```python
from build123d import *

# Parameters (mm, degrees)
ESQUISSE1_R                               = 30
BOSS_EXTRU_1_DEPTH                        = 5
ESQUISSE6_R                               = 35
ESQUISSE6_R_2                             = 30
BOSS_EXTRU_6_DEPTH                        = 5
ESQUISSE7_R                               = 32.5
ESQUISSE7_R_2                             = 30
BOSS_EXTRU_8_DEPTH                        = 35
CONG_2_R                                  = 10
BOSS_EXTRU_9_DEPTH                        = 30
BOSS_EXTRU_10_DEPTH                       = 12
CHANFREIN1_SIZE                           = 6
CONG_3_R                                  = 5
ENL_V_MAT_EXTRU_1_REACH                   = 89.234
ENL_V_MAT_EXTRU_1_END_RADIUS              = 32.5
ESQUISSE10_R                              = 4.5
ESQUISSE11_R                              = 4.5
ESQUISSE11_R_2                            = 2.6
BOSS_EXTRU_11_DEPTH                       = 3
R_P_TITION_CIRCULAIRE1_COUNT              = 4
CHANFREIN1_OF_R_P_TITION_CIRCULAIRE1_SIZE = 6


# Some blends are built 0.0001 mm under size
with BuildPart() as part:
    # Esquisse1 → Boss.-Extru.1 (new body)
    with BuildSketch(Plane.XY):
        with BuildLine():
            Line((-45.620718977, 15), (-70, 15))
            Line((-70, 15), (-70, -15))
            Line((-70, -15), (-45.620718977, -15))
            ThreePointArc((-45.620718977, -15), (-36.774201608, -17.062911874), (-29.752642811, -22.826086957))
            ThreePointArc((-29.752642811, -22.826086957), (37.5, 0), (-29.752642811, 22.826086957))
            ThreePointArc((-29.752642811, 22.826086957), (-36.774201608, 17.062911874), (-45.620718977, 15))
        make_face()
        Circle(ESQUISSE1_R, mode=Mode.SUBTRACT)
    extrude(amount=BOSS_EXTRU_1_DEPTH)

    # Esquisse6 → Boss.-Extru.6 (add)
    with BuildSketch(Plane.XY.offset(5)):
        Circle(ESQUISSE6_R)
        Circle(ESQUISSE6_R_2, mode=Mode.SUBTRACT)
    extrude(amount=BOSS_EXTRU_6_DEPTH)

    # Esquisse7 → Boss.-Extru.8 (add)
    with BuildSketch(Plane.XY.offset(10)):
        Circle(ESQUISSE7_R)
        Circle(ESQUISSE7_R_2, mode=Mode.SUBTRACT)
    extrude(amount=BOSS_EXTRU_8_DEPTH)

    # Congé2
    # the kernel refuses this fillet: 10 mm, written as the material it adds along each edge
    with BuildSketch(Plane(origin=(0, 0, 10), x_dir=(1, 0, 0), z_dir=(0, -1, 0))) as cong_2_piece_1:
        with BuildLine():
            CenterArc((42.5, 6.614378278), CONG_2_R, 180, 41.409622109)
            Line((32.5, 6.614378278), (32.3, 6.614378278))
            Line((32.3, 6.614378278), (32.3, 0))
            Line((32.3, 0), (32.5, -0.2))
            ThreePointArc((32.5, -0.2), (33.75, -0.2), (34.85, -0.132287566))
            Line((34.85, -0.132287566), (35, 0))
        make_face()
    revolve(axis=Axis((0, 0, 10), (0, 0, 1)))

    # Esquisse8 → Boss.-Extru.9 (add)
    with BuildSketch(Plane.XY.offset(5)):
        with BuildLine():
            Line((-70, -15), (-70, 15))
            Line((-70, 15), (-43.874821937, 15))
            ThreePointArc((-43.874821937, 15), (-39.966142137, 13.118047822), (-38.999841722, 8.888888889))
            ThreePointArc((-38.999841722, 8.888888889), (-40, 0), (-38.999841722, -8.888888889))
            ThreePointArc((-38.999841722, -8.888888889), (-39.966142137, -13.118047822), (-43.874821937, -15))
            Line((-43.874821937, -15), (-70, -15))
        make_face()
    extrude(amount=BOSS_EXTRU_9_DEPTH)

    # Esquisse9 → Boss.-Extru.10 (add)
    with BuildSketch(Plane.XY.offset(45)):
        Polygon((-32.405891584, -2.471475398), (-29.300063043, -14.062585313), (-21.572656433, -11.992032952), (-24.678484974, -0.400923037), align=None)
    boss_extru_10 = extrude(amount=-BOSS_EXTRU_10_DEPTH)

    # Chanfrein1
    # the kernel refuses this chamfer: 6 mm, written as the material it adds along each edge
    with BuildSketch(Plane(origin=(0, 0, 33), x_dir=(-0.5590908430517356, -0.8291064040373223, 0), z_dir=(0.8291064040373223, -0.5590908430517356, 0))) as chanfrein1_piece_1_section:
        Polygon((30, CHANFREIN1_SIZE), (30 - CHANFREIN1_SIZE, 0), (30, 0), align=None)
    chanfrein1_piece_1 = revolve(axis=Axis((0, 0, 33), (0, 0, -1)), revolution_arc=82.01410645, mode=Mode.PRIVATE)
    chanfrein1_piece_1 = split(chanfrein1_piece_1, bisect_by=Plane(origin=(-25.327272202, -12.998079215, 31.008979001), z_dir=(-0.25881904510251486, 0.96592582628907, 0)), keep=Keep.TOP, mode=Mode.PRIVATE)
    chanfrein1_piece_1 = split(chanfrein1_piece_1, bisect_by=Plane(origin=(-28.433100743, -1.4069693, 31.008979001), z_dir=(0.2588190451025147, -0.96592582628907, 0)), keep=Keep.TOP, mode=Mode.PRIVATE)
    chanfrein1_piece_1 = split(chanfrein1_piece_1, bisect_by=Plane(origin=(-23.125570703, -6.196477994, 31.008979001), z_dir=(-0.9659258262890699, -0.2588190451025148, 0)), keep=Keep.TOP, mode=Mode.PRIVATE)
    add(chanfrein1_piece_1)

    # Congé3
    cong_3_edges = [part.edges().sort_by_distance(p)[0] for p in [
        (37.5, 0, 0),
        (-57.810359489, 15, 0),
        (-57.810359489, -15, 0),
        (-36.774201608, -17.062911874, 0),
        (-36.774201608, 17.062911874, 0),
    ]]
    fillet(cong_3_edges, radius=CONG_3_R - 0.0001)  # a hair under: the kernel refuses the full size

    # Enlèv. mat.-Extru.1: up to this cylinder (the profile starts inside it)
    enl_v_mat_extru_1_end = Plane(origin=(0, 0, 39), z_dir=(0, 0, -1)) * Cylinder(ENL_V_MAT_EXTRU_1_END_RADIUS, 244.468, mode=Mode.PRIVATE)
    # Esquisse10 → Enlèv. mat.-Extru.1 (cut, up to the surface)
    with BuildSketch(Plane(origin=(-23.125570703, -6.196477994, 0), x_dir=(0, 0, -1), z_dir=(0.96592582628907, 0.25881904510251497, 0)), mode=Mode.PRIVATE) as enl_v_mat_extru_1_sk1:
        with Locations(Location((-39, 0, 0), (0, 0, 90))):
            Circle(ESQUISSE10_R)
    enl_v_mat_extru_1_tool1 = extrude(enl_v_mat_extru_1_sk1.sketch, amount=-ENL_V_MAT_EXTRU_1_REACH, mode=Mode.PRIVATE) & enl_v_mat_extru_1_end
    enl_v_mat_extru_1 = enl_v_mat_extru_1_tool1.solids().sort_by_distance((-23.125571, -6.196478, 39))[0]
    add(enl_v_mat_extru_1, mode=Mode.SUBTRACT)

    # Esquisse11 → Boss.-Extru.11 (add)
    with BuildSketch(Plane(origin=(-23.125570703, -6.196477994, 0), x_dir=(0, 0, -1), z_dir=(0.96592582628907, 0.25881904510251497, 0))):
        with Locations(Location((-39, 0, 0), (0, 0, 90))):
            Circle(ESQUISSE11_R)
        with Locations(Location((-39, 0, 0), (0, 0, 90))):
            Circle(ESQUISSE11_R_2, mode=Mode.SUBTRACT)
    boss_extru_11 = extrude(amount=-BOSS_EXTRU_11_DEPTH)

    # Répétition circulaire1: Boss.-Extru.10, Enlèv. mat.-Extru.1, Boss.-Extru.11 ×4 about axis
    r_p_tition_circulaire1_axis = Axis((0, 0, 0), (0, 0, 1))
    add([boss_extru_10.rotate(r_p_tition_circulaire1_axis, i * 360 / R_P_TITION_CIRCULAIRE1_COUNT) for i in range(1, R_P_TITION_CIRCULAIRE1_COUNT)])
    add([enl_v_mat_extru_1.rotate(r_p_tition_circulaire1_axis, i * 360 / R_P_TITION_CIRCULAIRE1_COUNT) for i in range(1, R_P_TITION_CIRCULAIRE1_COUNT)], mode=Mode.SUBTRACT)
    add([boss_extru_11.rotate(r_p_tition_circulaire1_axis, i * 360 / R_P_TITION_CIRCULAIRE1_COUNT) for i in range(1, R_P_TITION_CIRCULAIRE1_COUNT)])

    # Chanfrein1 of Répétition circulaire1
    # the kernel refuses this chamfer: 6 mm, written as the material it adds along each edge
    with BuildSketch(Plane(origin=(0, 0, 33), x_dir=(0.8291064040373222, -0.559090843051736, 0), z_dir=(0.559090843051736, 0.8291064040373222, 0))) as chanfrein1_of_r_p_tition_circulaire1_piece_1_section:
        Polygon((30, CHANFREIN1_OF_R_P_TITION_CIRCULAIRE1_SIZE), (30 - CHANFREIN1_OF_R_P_TITION_CIRCULAIRE1_SIZE, 0), (30, 0), align=None)
    chanfrein1_of_r_p_tition_circulaire1_piece_1 = revolve(axis=Axis((0, 0, 33), (0, 0, -1)), revolution_arc=82.01410645, mode=Mode.PRIVATE)
    chanfrein1_of_r_p_tition_circulaire1_piece_1 = split(chanfrein1_of_r_p_tition_circulaire1_piece_1, bisect_by=Plane(origin=(12.998079215, -25.327272202, 31.008979001), z_dir=(-0.96592582628907, -0.25881904510251474, 0)), keep=Keep.TOP, mode=Mode.PRIVATE)
    chanfrein1_of_r_p_tition_circulaire1_piece_1 = split(chanfrein1_of_r_p_tition_circulaire1_piece_1, bisect_by=Plane(origin=(1.4069693, -28.433100743, 31.008979001), z_dir=(0.96592582628907, 0.2588190451025146, 0)), keep=Keep.TOP, mode=Mode.PRIVATE)
    chanfrein1_of_r_p_tition_circulaire1_piece_1 = split(chanfrein1_of_r_p_tition_circulaire1_piece_1, bisect_by=Plane(origin=(6.196477994, -23.125570703, 31.008979001), z_dir=(0.25881904510251474, -0.9659258262890701, 0)), keep=Keep.TOP, mode=Mode.PRIVATE)
    add(chanfrein1_of_r_p_tition_circulaire1_piece_1)
    with BuildSketch(Plane(origin=(0, 0, 33), x_dir=(0.5590908430517355, 0.8291064040373223, 0), z_dir=(-0.8291064040373223, 0.5590908430517355, 0))) as chanfrein1_of_r_p_tition_circulaire1_piece_2_section:
        Polygon((30, CHANFREIN1_OF_R_P_TITION_CIRCULAIRE1_SIZE), (30 - CHANFREIN1_OF_R_P_TITION_CIRCULAIRE1_SIZE, 0), (30, 0), align=None)
    chanfrein1_of_r_p_tition_circulaire1_piece_2 = revolve(axis=Axis((0, 0, 33), (0, 0, -1)), revolution_arc=82.01410645, mode=Mode.PRIVATE)
    chanfrein1_of_r_p_tition_circulaire1_piece_2 = split(chanfrein1_of_r_p_tition_circulaire1_piece_2, bisect_by=Plane(origin=(25.327272202, 12.998079215, 31.008979001), z_dir=(0.25881904510251474, -0.96592582628907, 0)), keep=Keep.TOP, mode=Mode.PRIVATE)
    chanfrein1_of_r_p_tition_circulaire1_piece_2 = split(chanfrein1_of_r_p_tition_circulaire1_piece_2, bisect_by=Plane(origin=(28.433100743, 1.4069693, 31.008979001), z_dir=(-0.2588190451025146, 0.96592582628907, 0)), keep=Keep.TOP, mode=Mode.PRIVATE)
    chanfrein1_of_r_p_tition_circulaire1_piece_2 = split(chanfrein1_of_r_p_tition_circulaire1_piece_2, bisect_by=Plane(origin=(23.125570703, 6.196477994, 31.008979001), z_dir=(0.9659258262890701, 0.25881904510251474, 0)), keep=Keep.TOP, mode=Mode.PRIVATE)
    add(chanfrein1_of_r_p_tition_circulaire1_piece_2)
    with BuildSketch(Plane(origin=(0, 0, 33), x_dir=(-0.8291064040373223, 0.5590908430517356, 0), z_dir=(-0.5590908430517356, -0.8291064040373223, 0))) as chanfrein1_of_r_p_tition_circulaire1_piece_3_section:
        Polygon((30, CHANFREIN1_OF_R_P_TITION_CIRCULAIRE1_SIZE), (30 - CHANFREIN1_OF_R_P_TITION_CIRCULAIRE1_SIZE, 0), (30, 0), align=None)
    chanfrein1_of_r_p_tition_circulaire1_piece_3 = revolve(axis=Axis((0, 0, 33), (0, 0, -1)), revolution_arc=82.01410645, mode=Mode.PRIVATE)
    chanfrein1_of_r_p_tition_circulaire1_piece_3 = split(chanfrein1_of_r_p_tition_circulaire1_piece_3, bisect_by=Plane(origin=(-12.998079215, 25.327272202, 31.008979001), z_dir=(0.9659258262890701, 0.25881904510251463, 0)), keep=Keep.TOP, mode=Mode.PRIVATE)
    chanfrein1_of_r_p_tition_circulaire1_piece_3 = split(chanfrein1_of_r_p_tition_circulaire1_piece_3, bisect_by=Plane(origin=(-1.4069693, 28.433100743, 31.008979001), z_dir=(-0.9659258262890701, -0.25881904510251447, 0)), keep=Keep.TOP, mode=Mode.PRIVATE)
    chanfrein1_of_r_p_tition_circulaire1_piece_3 = split(chanfrein1_of_r_p_tition_circulaire1_piece_3, bisect_by=Plane(origin=(-6.196477994, 23.125570703, 31.008979001), z_dir=(-0.2588190451025146, 0.96592582628907, 0)), keep=Keep.TOP, mode=Mode.PRIVATE)
    add(chanfrein1_of_r_p_tition_circulaire1_piece_3)


solid = part.part
```
Geometry check sheet. Reference: the model listing, model coordinates, mm. A direction names the side the tool comes from. Coordinates: 2 decimals unless noted, no trailing zeros. Order: outer loops, then holes, each group sorted by start corner. A loop starts at its lowest first (then second) coordinate and runs counter-clockwise, first axis right, second up. Notation, with made-up numbers: M -16.5,-21 L 9.5,-21 A19 ccw 9.5,14 Z; hole C -38,33 d4. An arc over 180 degrees is marked long. Answer as a JSON object with one key per item and string values.
Q1. Release check for a two-part mould opening along Y. For faces 1 (the cylindrical face through (-58, 13, 1)), 2 (the cylindrical face through (-25.79, -19.78, 30.61)), 3 (the cylindrical face through (-7.12, 24.41, 36.46)) record: released by +Y, released by -Y, zero draft, split by the parting line, or undercut.
Results are:
{"face 1": "released by +Y", "face 2": "split by the parting line", "face 3": "undercut"}
Q2. Depth check by flat-ended pin: pin 1 Ø1 at (x, z) = (-56.5, 30.5) entering from -Y; pin 2 Ø5 at (x, z) = (-40.5, 16.5) entering from -Y; pin 3 Ø1.5 at (x, y) = (-43.5, 14) entering from -Z. Enter the tip coordinate at first touch or a pass-through.
Results are:
{"pin 1": "stops at y = -15", "pin 2": "stops at y = -14.92", "pin 3": "stops at z = 1.11"}
Q3. Cross-section at A-A on z = 25. Record the cut outline in (x, y), and give its area (3 significant figures).
Results are:
{"outline": "M -70,-15 L -43.87,-15 A5 ccw -39,-8.89 A40 cw -39,8.89 A5 ccw -43.87,15 L -70,15 Z; C 0,0 d65; hole C 0,0 d60", "area": "1,400 mm²"}
Q4. Tool access check on faces 4 (the flat face through (-26.783, -4.136, 39.063)), 5 (the conical face through (-7.067, 26.015, 30.042)), 6 (the cylindrical face through (-58, -13, 1)), 7 (the flat face through (-54, 0, 35)). Record the directions out of +Z, -Z, +X, -X, +Y, -Y that give a thin tool (end or side, any length) a straight path to the whole face; none if there is none.
Results are:
{"face 4": "none", "face 5": "-Z", "face 6": "-Z, -X, -Y", "face 7": "+Z, -X, +Y, -Y"}
Q5. Scan lines: line 1 (X direction, y = 0, z = 25); line 2 (Y direction, x = -9, z = 24); line 3 (Z direction, x = -34.5, y = 8). Record each from-to range of solid material in increasing order.
Results are:
{"line 1": "x = -70 to -40, -32.5 to -30, 30 to 32.5", "line 2": "y = -31.23 to -28.62, 28.62 to 31.23", "line 3": "z = 0 to 5"}
Q6. Cross-section at C-C on z = 14. Record the cut outline in (x, y), and give its area (3 significant figures).
Results are:
{"outline": "M -70,-15 L -43.87,-15 A5 ccw -39,-8.89 A40 cw -39,8.89 A5 ccw -43.87,15 L -70,15 Z; C 0,0 d65.7; hole C 0,0 d60", "area": "1,470 mm²"}
Q7. Cross-section at B-B on x = -52.5. Record the cut outline in (y, z), and give its area (3 significant figures).
Results are:
{"outline": "M -15,5 A5 ccw -10,0 L 10,0 A5 ccw 15,5 L 15,35 L -15,35 Z", "area": "1,040 mm²"}
